Here's the drawing with two shaded views (mm, measured from the low corner). I have some questions. Give positions to 0.01 mm unless a question says otherwise; leave off trailing zeros. Write each loop counter-clockwise with the first axis right and the second up, starting at its lowest first coordinate (ties: lowest second). Pieces come first, ordered by that corner, then holes. Notation, with made-up numbers: (70.25, 89.5) -> (125.25, 89.5) arc R32 cw to (125.25, 127.5) -> close; hole circle Ø5 at (35.5, 17). An arc over 180 degrees is marked (long way). One line per question, with ' | ' between items.
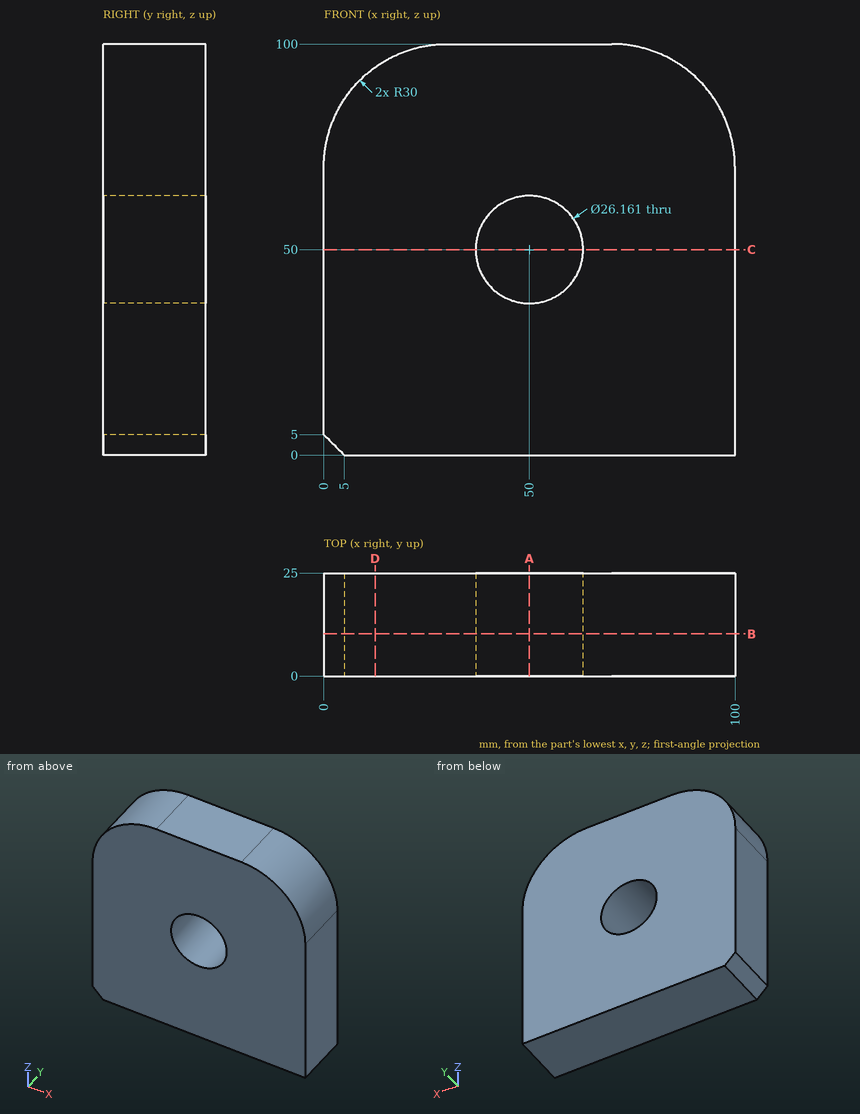
Q1. Will this pin go through, and if not, where does the flat tip stop? pin 1 (12 mm diameter, centred on x = 15, y = 6.5, fed in from +Z).
Answer below:
pin 1: stops at z = 98.62
Q2. Imagine slicing it at A-A on x = 50. Please give me the cut outline in (y, z), and give its area (3 significant figures).
Answer below:
outline: (0, 0) -> (25, 0) -> (25, 36.92) -> (0, 36.92) -> close; (0, 63.08) -> (25, 63.08) -> (25, 100) -> (0, 100) -> close | area: 1,850 mm^2
Q3. Imagine slicing it at B-B on y = 10.25. Please give me the cut outline in (x, z).
Answer below:
outline: (0, 5) -> (5, 0) -> (100, 0) -> (100, 70) arc R30 ccw to (70, 100) -> (30, 100) arc R30 ccw to (0, 70) -> close; hole circle Ø26.16 at (50, 50)
Q4. If I drill on line 1 along Z through (x, y) = (50, 7.5); line 2 along X through (y, z) = (5.75, 53.5); line 3 along Z through (x, y) = (22, 8), over which ranges is the centre line in solid material (lowest first)?
Answer below:
line 1: z = 0 to 36.92, 63.08 to 100 | line 2: x = 0 to 37.4, 62.6 to 100 | line 3: z = 0 to 98.91
Q5. Imagine slicing it at D-D on x = 12.5. Please give me the cut outline in (y, z), and give its area (3 significant figures).
Answer below:
outline: (0, 0) -> (25, 0) -> (25, 94.37) -> (0, 94.37) -> close | area: 2,360 mm^2
Q6. Imagine slicing it at C-C on z = 50. Please give me the cut outline in (x, y).
Answer below:
outline: (0, 0) -> (36.92, 0) -> (36.92, 25) -> (0, 25) -> close; (63.08, 0) -> (100, 0) -> (100, 25) -> (63.08, 25) -> close
